Design review of the part built by this model. Coordinates are the model's own, in mm. Face numbers are marked on the shaded views. Round coordinates to 2 decimals unless told otherwise and drop trailing zeros. Order: outer loops, then holes, each group sorted by start corner. A loop starts at its lowest first (then second) coordinate and runs counter-clockwise, first axis right, second up. Notation, with made-up numbers: (23.5, -28) - (72.5, -28) arc R15 cw to (72.5, -7) - close; hole circle Ø7 at (3.25, -8.5). An arc over 180 degrees is marked (long way). Write item = value, one per line.
Autodesk Inventor part; units mm, degrees
ref_plane "YZ Plane" through (0, 0, 0) normal (1, 0, 0) x (0, 1, 0)
ref_plane "XZ Plane" through (0, 0, 0) normal (0, 1, 0) x (-1, 0, 0)
ref_plane "XY Plane" through (0, 0, 0) normal (0, 0, 1) x (1, 0, 0)
sketch "Sketch1" plane through (0, 0, 0) normal (0, 0, 1) x (1, 0, 0)
  line L0 (-13, -4) -> (13, -4)
  line L1 (13, -4) -> (13, 4)
  line L2 (13, 4) -> (-13, 4)
  line L3 (-13, 4) -> (-13, -4)
  line L4 (-13, -4) -> (13, 4) construction
  line L5 (13, -4) -> (-13, 4) construction
  point P0 (0, 0)
  dimension "d0" = 26
  dimension "d1" = 8
extrude "Extrusion1" add sketch "Sketch1" along normal blind 7
sketch "Sketch2" plane through (0, 0, 7) normal (0, 0, 1) x (1, 0, 0)
  line L0 (0, 5.6) -> (0, -5.6)
  circle A0 centre (-7.5, 0) radius 1.75
  circle A1 centre (7.5, 0) radius 1.75
  line L1 (-18.2, 0) -> (18.2, 0)
  point P0 (0, 0)
  dimension "d4" = 3.5
  dimension "d5" = 15
extrude "Extrusion2" cut sketch "Sketch2" against normal through all
fillet "Fillet1" radius 2 4 edges at (-13, 4, 3.5) (-13, -4, 3.5) (13, -4, 3.5) (13, 4, 3.5)
properties part number "30_Lasercable_holder_B"
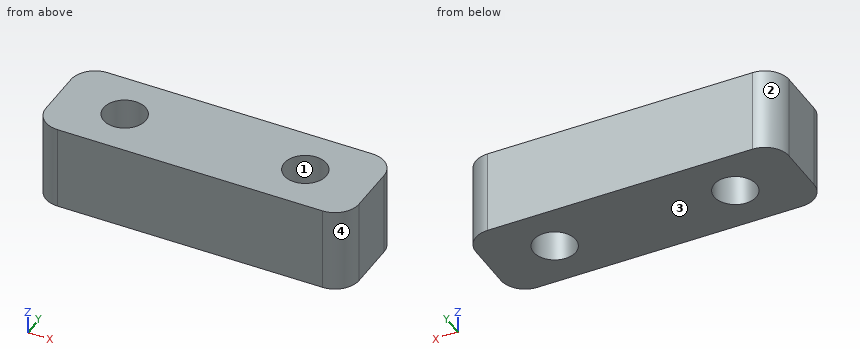
Item 1: The part is to be moulded in two halves that separate along X. For the marked faces 1, 2, 3 and 4, say which applies: +X half, -X half, draft (parallel to the pull), parting line (faces both ways), or undercut.
Data:
face_1 = undercut
face_2 = -X half
face_3 = draft
face_4 = +X half
Item 2: Take a section at A-A, the plane y = 0. State the section outline as (x, z) points.
Data:
outline = (-13, 0) - (-9.25, 0) - (-9.25, 7) - (-13, 7) - close; (-5.75, 0) - (5.75, 0) - (5.75, 7) - (-5.75, 7) - close; (9.25, 0) - (13, 0) - (13, 7) - (9.25, 7) - close
Item 3: Take a section at C-C, the plane z = 2.25. State the section outline as (x, y) points.
Data:
outline = (-13, -2) arc R2 ccw to (-11, -4) - (11, -4) arc R2 ccw to (13, -2) - (13, 2) arc R2 ccw to (11, 4) - (-11, 4) arc R2 ccw to (-13, 2) - close; hole circle Ø3.5 at (-7.5, 0); hole circle Ø3.5 at (7.5, 0)
Item 4: Take a section at B-B, the plane x = -7.5. State the section outline as (y, z) points, and give its area (3 significant figures).
Data:
outline = (-4, 0) - (-1.75, 0) - (-1.75, 7) - (-4, 7) - close; (1.75, 0) - (4, 0) - (4, 7) - (1.75, 7) - close
area = 31.5 mm2
Item 5: Take a section at D-D, the plane y = -1.5. State the section outline as (x, z) points, and give its area (3 significant figures).
Data:
outline = (-13, 0) - (-8.4, 0) - (-8.4, 7) - (-13, 7) - close; (-6.6, 0) - (6.6, 0) - (6.6, 7) - (-6.6, 7) - close; (8.4, 0) - (13, 0) - (13, 7) - (8.4, 7) - close
area = 157 mm2
Item 6: For line 1 along X through (y, z) = (0, 1.5); line 2 along Y through (x, z) = (7.5, 2.75); line 3 along X through (y, z) = (0.75, 3.25), list the stretches that pass through material, from the lowest coordinate up. Write a range as [from, to].
Data:
line_1 = [-13, -9.25], [-5.75, 5.75], [9.25, 13]
line_2 = [-4, -1.75], [1.75, 4]
line_3 = [-13, -9.08], [-5.92, 5.92], [9.08, 13]
